```python
from build123d import *

# Parameters (mm, degrees)
F0_R     = 50.8
F1_DEPTH = 91.44
F1_TAPER = 25
F2_R     = 38.1
F3_DEPTH = 25.4
F4_R     = 4.2924717139
F5_SIZE  = 17.78
F6_DEPTH = 106.172
F7_SIZE  = 11.938


with BuildPart() as f1:
    # F0 (on Front) → F1 (new body)
    with BuildSketch(Plane.XZ):
        Circle(F0_R)
    extrude(amount=F1_DEPTH, taper=F1_TAPER)

    # F2 (on face) → F3 (cut)
    with BuildSketch(Plane(origin=(0, 0, 0), x_dir=(-1, 0, 0), z_dir=(0, 1, 0))):
        Circle(F2_R)
    extrude(amount=-F3_DEPTH, mode=Mode.SUBTRACT)

    # F4
    f4_edges = [f1.edges().sort_by_distance(p)[0] for p in [
        (-50.8, 0, 0),
        (38.1, 0, 0),
    ]]
    fillet(f4_edges, radius=F4_R)

    # F5
    f5_edges = [f1.edges().sort_by_distance(p)[0] for p in [
        (38.1, -4.292472, 0),
        (38.1, -25.4, 0),
    ]]
    chamfer(f5_edges, length=F5_SIZE)

    # F6 (cut): a face of the model
    f6_faces = [f1.faces().sort_by_distance(p)[0] for p in [
        (0, -91.44, 0),
    ]]
    extrude(f6_faces, amount=-F6_DEPTH, mode=Mode.SUBTRACT)

    # F7
    f7_edges = [f1.edges().sort_by_distance(p)[0] for p in [
        (-8.160828, -25.4, 0),
    ]]
    chamfer(f7_edges, length=F7_SIZE)


solid = f1.part
```
Here's how the part is built. I have some questions about the finished solid (model axes, mm). A direction names the side the tool comes from. Give positions to 0.01 mm unless a question says otherwise; leave off trailing zeros. Order: outer loops, then holes, each group sorted by start corner. A loop starts at its lowest first (then second) coordinate and runs counter-clockwise, first axis right, second up. Notation, with made-up numbers: (71, -8) -> (107, -8) arc R29 cw to (107, 15) -> close; hole circle Ø7 at (43, 53). An arc over 180 degrees is marked (long way). Use CSV: the item, a comma, the result in double quotes. Start each with the question number.
Item 1: On a 3-axis mill with a long thin cutter (end or side, diameter ignored), from which of +Z, -Z, +X, -X, +Y, -Y can I reach the whole of each face in a straight line? I mean faces 1 (the cylindrical face through (30.235, -5.933, -23.183)), 2 (the cylindrical face through (7.784, -64.768, -2.451)). Say none if no direction works.
Item 2: Thinking about a two-plate mould opening in Z: for faces 3 (the flat face through (-23, 0, 36)), 4 (the conical face through (2.76, -24.54, 21)), 5 (the conical face through (-5.063, -58.852, -22.801)), 6 (the conical face through (-6.9, -36.8, -5.3)), which applies, pulls with the +Z half, pulls with the -Z half, needs draft (parallel to the pull), parting line crosses it, or undercut?
Item 3: If I drill on probe 1 along Z at (x, y) = (8.5, -16.5); probe 2 along X at (y, z) = (-14.5, -24); probe 3 along X at (y, z) = (-9.5, 26), over which ranges is the centre line in solid material (lowest first)? Write a range as [from, to].
Item 4: Suppose I cut it at B-B (y = -48.5). List the corners of the cut face in (x, z) for me, and give its area (3 significant figures).
Item 5: Suppose I cut it at C-C (y = -66). List the corners of the cut face in (x, z) for me.
Item 6: Suppose I cut it at A-A (x = 0). List the corners of the cut face in (y, z) for me.
Item 7: I'm going to push flat-ended pins straight in: P1, Ø3, axis at x = 20.5, z = 9.5, coming from the +Y side; P2, Ø2, axis at y = -32, z = 0.5, coming from the +X side; P3, Ø5, axis at x = 4.5, z = -13.5, coming from the +Y side. Where does each tip first touch, or does it pass through?
Answer block:
1,face 1,"+Y"
1,face 2,"+Y, -Y"
2,face 3,"needs draft"
2,face 4,"undercut"
2,face 5,"parting line crosses it"
2,face 6,"undercut"
3,probe 1,"z = [-42.26, -27.96], [27.96, 42.26]"
3,probe 2,"x = [-36.92, -19.97], [19.97, 36.92]"
3,probe 3,"x = [-38.4, -25.22], [25.22, 38.4]"
4,outline,"circle Ø56.37 at (0, 0); hole circle Ø16.32 at (0, 0)"
4,area,"2,290 mm^2"
5,outline,"circle Ø40.05 at (0, 0); hole circle Ø16.32 at (0, 0)"
6,outline,"(-91.44, -8.16) -> (-6.11, -47.95) arc R4.29 ccw to (0, -44.06) -> (0, -42.39) arc R4.29 ccw to (-4.29, -38.1) -> (-7.62, -38.1) -> (-25.4, -20.32) -> (-25.4, -20.1) -> (-37.34, -8.16) -> close; (-91.44, 8.16) -> (-37.34, 8.16) -> (-25.4, 20.1) -> (-25.4, 20.32) -> (-7.62, 38.1) -> (-4.29, 38.1) arc R4.29 ccw to (0, 42.39) -> (0, 44.06) arc R4.29 ccw to (-6.11, 47.95) -> close"
7,P1,"stops at y = -21.63"
7,P2,"stops at x = 36.34"
7,P3,"stops at y = -28.77"
